Work out the finished part from the listing and answer in its coordinate system (mm). A direction names the side the tool comes from. Round coordinates to 2 decimals unless told otherwise and drop trailing zeros. Write each loop counter-clockwise with the first axis right and the second up, starting at its lowest first coordinate (ties: lowest second). Pieces come first, ordered by that corner, then holes. Notation, with made-up numbers: M -32.5,1 L -20.5,1 A12 cw -20.5,19 Z; hole C 86,8.25 d8. An arc over 180 degrees is marked long. Answer in a Markdown table with one row per item.
Autodesk Inventor part; units mm, degrees
ref_plane "YZ Plane" through (0, 0, 0) normal (1, 0, 0) x (0, 1, 0)
ref_plane "XZ Plane" through (0, 0, 0) normal (0, 1, 0) x (-1, 0, 0)
ref_plane "XY Plane" through (0, 0, 0) normal (0, 0, 1) x (1, 0, 0)
sketch "Sketch1" plane through (0, 0, 0) normal (0, 1, 0) x (-1, 0, 0)
  circle A0 centre (53.5305, 0) radius 2.3813
  circle A1 centre (0, -53.5305) radius 2.3876
  circle A2 centre (-53.5305, 0) radius 2.3876
  circle A3 centre (0, 53.5305) radius 2.3876
  line L0 (0, 60.2361) -> (-6.35, 60.2361)
  line L1 (-6.35, 60.2361) -> (6.35, 60.2361)
  line L2 (6.35, 60.2361) -> (6.35, 48.8011)
  line L3 (-6.35, 60.2361) -> (-6.35, 48.8011)
  line L4 (-60.2361, 0) -> (-60.2361, -6.35)
  line L5 (-60.2361, -6.35) -> (-60.2361, 6.35)
  line L6 (-60.2361, 6.35) -> (-48.8011, 6.35)
  line L7 (-60.2361, -6.35) -> (-48.8011, -6.35)
  line L8 (0, -60.2361) -> (-6.35, -60.2361)
  line L9 (-6.35, -60.2361) -> (6.35, -60.2361)
  line L10 (6.35, -60.2361) -> (6.35, -48.8011)
  line L11 (-6.35, -60.2361) -> (-6.35, -48.8011)
  line L12 (60.2361, 0) -> (60.2361, -6.35)
  line L13 (60.2361, -6.35) -> (60.2361, 6.35)
  line L14 (60.2361, 6.35) -> (48.8011, 6.35)
  line L15 (60.2361, -6.35) -> (48.8011, -6.35)
  arc A4 (6.35, -48.8011) -> (48.8011, -6.35) centre (0, 0) ccw
  arc A5 (-48.8011, -6.35) -> (-6.35, -48.8011) centre (0, 0) ccw
  arc A6 (48.8011, 6.35) -> (6.35, 48.8011) centre (0, 0) ccw
  arc A7 (-6.35, 48.8011) -> (-48.8011, 6.35) centre (0, 0) ccw
  circle A8 centre (0, 0) radius 49.2125
  dimension "d6" = 4.7625
  dimension "d7" = 4.7752
  dimension "d8" = 4.7752
  dimension "d9" = 4.7752
  dimension "d11" = 6.7056
  dimension "d12" = 6.7056
  dimension "d13" = 6.7056
  dimension "d14" = 6.7056
  dimension "d15" = 6.35
  dimension "d16" = 12.7
  dimension "d17" = 6.35
  dimension "d18" = 12.7
  dimension "d19" = 6.35
  dimension "d20" = 12.7
  dimension "d21" = 6.35
  dimension "d22" = 12.7
extrude "Extrusion1" add sketch "Sketch1" along normal blind 3.175
sketch "Sketch2" plane through (0, 3.175, 0) normal (0, 1, 0) x (1, 0, 0)
  arc A0 (48.8011, 6.35) -> (6.35, 48.8011) centre (0, 0) ccw
  arc A1 (-48.8011, -6.35) -> (-6.35, -48.8011) centre (0, 0) ccw
  circle A2 centre (0, 0) radius 49.2125
extrude "Extrusion2" add sketch "Sketch2" along normal blind 35.7188
sketch "Sketch3" plane through (0, 38.8937, 0) normal (0, 1, 0) x (1, 0, 0)
  circle A0 centre (0, 0) radius 49.2125
  circle A1 centre (0, 0) radius 6.35
  dimension "d27" = 12.7
extrude "Extrusion3" add sketch "Sketch3" along normal blind 3.175 contours A1
sketch "Sketch4" plane through (0, 42.0688, 0) normal (0, 1, 0) x (1, 0, 0)
  circle A0 centre (0, 0) radius 6.35
  circle A1 centre (0, 0) radius 49.2125
  dimension "d30" = 98.425
extrude "Extrusion4" add sketch "Sketch4" along normal blind 3.9688 contours A0 | A1
properties part number "Rotating Base"
1. Determine the mould class of faces 4 (the flat face through (-56, 3.175, 2)), 5 (the flat face through (6.35, 2, -55)), 6 (the cylindrical face through (-51.15, 1.57, -0.1)), 7 (the cylindrical face through (51.253, 1.565, -0.717)) for opening direction X: released by +X, released by -X, zero draft, split by the parting line, or undercut.
Calculated:
| item | result |
|---|---|
| face 4 | zero draft |
| face 5 | released by +X |
| face 6 | undercut |
| face 7 | undercut |
2. The part is cut by section A-A (z = 0). Count the separate pieces of the cut face and the enclosed holes in it, plus the area to 3 significant figures.
Calculated:
| item | result |
|---|---|
| separate pieces | 3 |
| enclosed holes | 0 |
| area | 4,300 mm² |
3. Given pin 1 (2.5 mm diameter, centred on x = 55, y = 2.5, fed in from -Z); pin 2 (5.5 mm diameter, centred on x = 0, z = 53.53, fed in from +Y) (3 decimals); pin 3 (1.5 mm diameter, centred on y = 29.5, z = -38, fed in from -X), each flat-ended and moving along its own axis, determine where each tip first touches the part or whether it passes through.
Calculated:
| item | result |
|---|---|
| pin 1 | stops at z = -6.35 |
| pin 2 | stops at y = 3.175 |
| pin 3 | stops at x = -32.16 |
4. A tool of negligible diameter and unlimited length cuts with its end or side. For faces 1 (the cylindrical face through (-1.38, 40.46, -6.2)), 2 (the flat face through (55, 2, -6.35)), 3 (the flat face through (-55, 2, -6.35)), from which of +Z, -Z, +X, -X, +Y, -Y can it reach the whole face along a straight path? Write none if from no direction.
Calculated:
| item | result |
|---|---|
| face 1 | none |
| face 2 | -Z, +X, +Y, -Y |
| face 3 | -Z, -X, +Y, -Y |
5. The part is cut by section D-D (z = 20). Determine the outline of the cut face in (x, y) (3 decimals), plus the area to 3 significant figures.
Calculated:
| item | result |
|---|---|
| outline | M -44.965,0 L 44.965,0 L 44.965,38.894 L -44.965,38.894 Z; M -44.965,42.069 L 44.965,42.069 L 44.965,46.038 L -44.965,46.038 Z |
| area | 3,850 mm² |
6. Consider line 1 along Z through (x, y) = (0, 2); line 2 along Y through (x, z) = (26, 1); line 3 along Z through (x, y) = (6.5, 30.5). Determine where each line is inside the solid, lowest interval first. Write a range as from..to.
Calculated:
| item | result |
|---|---|
| line 1 | z = -60.24..-55.92, -51.14..51.14, 55.92..60.24 |
| line 2 | y = 0..38.89, 42.07..46.04 |
| line 3 | z = -48.78..48.78 |
7. The part is cut by section C-C (x = -46). Determine the outline of the cut face in (y, z) (3 decimals).
Calculated:
| item | result |
|---|---|
| outline | M 0,-17.489 L 38.894,-17.489 L 38.894,17.489 L 0,17.489 Z; M 42.069,-17.489 L 46.038,-17.489 L 46.038,17.489 L 42.069,17.489 Z |
